Source: CAD feature listing. Evaluate the final solid. Frame: model axes, mm. A direction names the side the tool comes from. Coordinates: 2 decimals unless noted, no trailing zeros. Order: outer loops, then holes, each group sorted by start corner. A loop starts at its lowest first (then second) coordinate and runs counter-clockwise, first axis right, second up.
```python
from build123d import *

# Parameters (mm, degrees)
F3_D     = 8.654
F3_DEPTH = 10
F3_TIP   = 2.5999238985
F4_R     = 5
F5_SIZE  = 1


with BuildPart() as f1:
    # F0 (on Front) → F1 (revolve)
    with BuildSketch(Plane.XZ):
        Polygon((15.0574529544, 30.9514049441), (0, 30.9514049441), (0, 25.9012449533), (3.761041211, 25.9012449533), (3.761041211, 8.42503272), (0, 8.42503272), (0, 5.7670525275), (10.4059893638, 5.7670525275), (10.4059893638, 8.42503272), (7.0835147053, 8.42503272), (7.0835147053, 25.9012449533), (15.0574529544, 25.9012449533), align=None)
    revolve(axis=Axis((5.2029946819, 0, 0), (1, 0, 0)))

    # F3
    with Locations(Plane(origin=(3.761041211, 0, 0), x_dir=(0, -1, 0), z_dir=(-1, 0, 0))):
        with Locations((-15.9109056188, 5.1697666204), (0, 16.7297162116), (15.9109056188, 5.1697666204), (9.8334804642, -13.5346247262), (-9.8334804642, -13.5346247262)):
            Hole(F3_D / 2, depth=F3_DEPTH)
            with Locations((0, 0, -(F3_DEPTH + F3_TIP / 2))):  # 118° drill point
                Cone(0, F3_D / 2, F3_TIP, mode=Mode.SUBTRACT)

    # F4
    f4_edges = [f1.edges().sort_by_distance(p)[0] for p in [
        (0, 0, -30.951405),
        (15.057453, 0, -30.951405),
    ]]
    fillet(f4_edges, radius=F4_R)

    # F5
    f5_edges = [f1.edges().sort_by_distance(p)[0] for p in [
        (0, 0, -8.425033),
        (0, 0, -5.767053),
        (7.083515, 4.327, 16.729716),
        (7.083515, 14.16048, -13.534625),
        (7.083515, -11.583906, 5.169767),
        (7.083515, -5.50648, -13.534625),
        (3.761041, 14.16048, -13.534625),
        (3.761041, 20.237906, 5.169767),
        (3.761041, 4.327, 16.729716),
        (3.761041, -5.50648, -13.534625),
        (3.761041, -11.583906, 5.169767),
    ]]
    chamfer(f5_edges, length=F5_SIZE)


solid = f1.part
```
1. Section query A-A, the plane y = 0. Count the separate pieces of the cut face and the enclosed holes in it, plus the area to 3 significant figures.
2. Access query for faces 1 (the flat face through (3.761, 0, 11)), 2 (the cylindrical face through (5.432, 2.326, 20.378)), 3 (the flat face through (10.406, 5, -4)). Directions: +Z, -Z, +X, -X, +Y, -Y. A direction counts if a zero-diameter tool reaches every point of the face in a straight line with its end or side. Return the directions, or none.
3. Contact query for flat-ended pins moving along their axis: P1, Ø1, axis at x = 12, y = -6, coming from the -Z side; P2, Ø1, axis at x = 11, y = -20, coming from the +Z side; P3, Ø3, axis at x = 12.5, y = 2, coming from the +Z side. Output: stop coordinate, or through.
4. Section query B-B, the plane x = 13.75. Output: boundary loops of the cut face in (y, z).
5. Material intervals for line 1 along Z through (x, y) = (5.15, 0); line 2 along Z through (x, y) = (9.5, 0); line 3 along Y through (x, z) = (5.75, -17), sorted ascending.
6. Draft query along Z for faces 4 (the cylindrical face through (2.361, -2.531, 8.036)), 5 (the cylindrical face through (8.721, -2.531, 8.036)), 6 (the cylindrical face through (7.493, 30.215, -6.71)), 7 (the flat face through (0, 6.6, 2.2)). Return one class per face: +Z half, -Z half, draft (parallel to the pull), parting line (faces both ways), or undercut.
Answer key:
1. separate pieces: 3
1. enclosed holes: 0
1. area: 269 mm2
2. face 1: -X
2. face 2: +X, -X
2. face 3: +X
3. P1: stops at z = -30.18
3. P2: stops at z = 23.94
3. P3: stops at z = 30.81
4. outline: circle Ø58.65 at (0, 0); hole circle Ø51.8 at (0, 0)
5. line 1: z = -30.95 to -5.77, 5.77 to 12.4, 21.06 to 30.95
5. line 2: z = -30.95 to -25.9, -8.43 to -5.77, 5.77 to 8.43, 25.9 to 30.95
5. line 3: y = -25.86 to -12.42, -7.24 to 7.24, 12.42 to 25.86
6. face 4: undercut
6. face 5: undercut
6. face 6: parting line
6. face 7: draft
